Autodesk Inventor part; units mm, degrees
ref_plane "YZ Plane" through (0, 0, 0) normal (1, 0, 0) x (0, 1, 0)
ref_plane "XZ Plane" through (0, 0, 0) normal (0, 1, 0) x (-1, 0, 0)
ref_plane "XY Plane" through (0, 0, 0) normal (0, 0, 1) x (1, 0, 0)
sketch "Sketch1" plane through (0, 0, 0) normal (0, 1, 0) x (-1, 0, 0)
  circle A0 centre (0, 0) radius 5
  dimension "d0" = 10
extrude "Extrusion1" add sketch "Sketch1" along normal blind 160
thread "Thread1"
sketch "Sketch2" plane through (0, 160, 0) normal (0, 1, 0) x (1, 0, 0)
  circle A0 centre (0, 0) radius 5
  circle A1 centre (0, 0) radius 10 construction
  line L0 (-10, 0) -> (-5, 8.6603)
  line L1 (-5, 8.6603) -> (5, 8.6603)
  line L2 (5, 8.6603) -> (10, 0)
  line L3 (10, 0) -> (5, -8.6603)
  line L4 (5, -8.6603) -> (-5, -8.6603)
  line L5 (-5, -8.6603) -> (-10, 0)
  dimension "d5" = 20
extrude "Extrusion2" add sketch "Sketch2" along normal blind 10 contours A0 | L0 L1 L2 L3 L4 L5
properties part number "BoltA" material "Titanium"
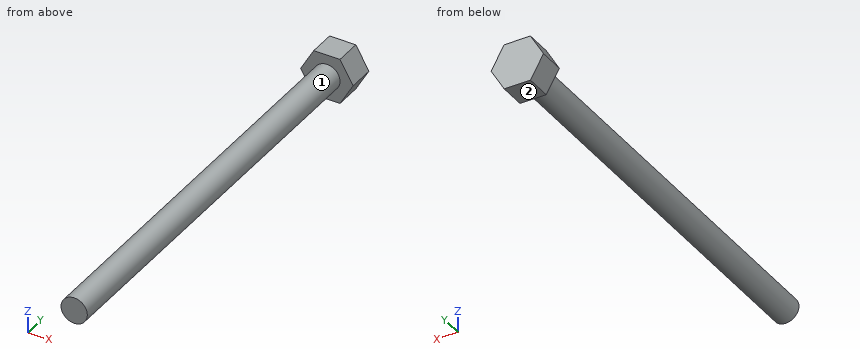
Input: part model. Units: mm. Frame: model coordinates. Face numbers are marked on the shaded views. A direction names the side the tool comes from. Coordinates: 2 decimals unless noted, no trailing zeros. Order: outer loops, then holes, each group sorted by start corner. A loop starts at its lowest first (then second) coordinate and runs counter-clockwise, first axis right, second up.
1. Cut plane C-C, the plane z = 2.75. Return loops of the section in (x, y), plus the area to 3 significant figures.
Checked values:
outline: (-8.41, 160) - (-4.18, 160) - (-4.18, 0) - (4.18, 0) - (4.18, 160) - (8.41, 160) - (8.41, 170) - (-8.41, 170) - close
area: 1,500 mm2
2. Contact query for flat-ended pins moving along their axis: P1, Ø1.5, axis at x = -1.5, y = 125.5, coming from the -Z side; P2, Ø8, axis at x = 6.5, y = 54, coming from the +Z side; P3, Ø3, axis at y = 26.5, z = 1.5, coming from the +X side. Output: stop coordinate, or through.
Checked values:
P1: stops at z = -4.94
P2: stops at z = 4.33
P3: stops at x = 5
3. Ray query, line 1 along Y through (x, z) = (-3.25, -7.25); line 2 along X through (y, z) = (34.5, 0.25); line 3 along Z through (x, y) = (3, 117.5). Return the intervals inside material, ascending.
Checked values:
line 1: y = 160 to 170
line 2: x = -4.99 to 4.99
line 3: z = -4 to 4
4. Cut plane D-D, the plane x = -6.5. Return loops of the section in (y, z), plus the area to 3 significant figures.
Checked values:
outline: (160, -6.06) - (170, -6.06) - (170, 6.06) - (160, 6.06) - close
area: 121 mm2
5. Cut plane A-A, the plane x = 0. Return loops of the section in (y, z), plus the area to 3 significant figures.
Checked values:
outline: (0, -5) - (160, -5) - (160, -8.66) - (170, -8.66) - (170, 8.66) - (160, 8.66) - (160, 5) - (0, 5) - close
area: 1,770 mm2
6. Access query for the marked faces 1 and 2. Directions: +Z, -Z, +X, -X, +Y, -Y. A direction counts if a zero-diameter tool reaches every point of the face in a straight line with its end or side. Return the directions, or none.
Checked values:
face 1: -Y
face 2: -Z, +X, -X, +Y, -Y
7. Cut plane B-B, the plane y = 120. Return loops of the section in (x, z).
Checked values:
outline: circle Ø10 at (0, 0)
